Autodesk Inventor part; units mm, degrees
ref_plane "YZ Plane" through (0, 0, 0) normal (1, 0, 0) x (0, 1, 0)
ref_plane "XZ Plane" through (0, 0, 0) normal (0, 1, 0) x (-1, 0, 0)
ref_plane "XY Plane" through (0, 0, 0) normal (0, 0, 1) x (1, 0, 0)
sketch "Sketch1" plane through (0, 0, 0) normal (0, 1, 0) x (-1, 0, 0)
  line L0 (-25, -30) -> (25, -30)
  line L1 (25, -30) -> (25, 30)
  line L2 (25, 30) -> (-25, 30)
  line L3 (-25, 30) -> (-25, -30)
  line L4 (-25, -30) -> (25, 30) construction
  line L5 (25, -30) -> (-25, 30) construction
  point P0 (0, 0)
  dimension "d0" = 50
  dimension "d1" = 60
extrude "Extrusion1" add sketch "Sketch1" along normal blind 53
sketch "Sketch2" plane through (-25, 0, 30) normal (0, 0, 1) x (1, 0, 0)
  line L0 (0, 0) -> (0, 53)
  line L1 (50, 0) -> (50, 53)
  line L2 (0, 53) -> (50, 53)
  line L3 (50, 53) -> (50, 49)
  line L4 (50, 49) -> (0, 49)
  line L5 (0, 49) -> (0, 53)
  line L6 (12.5, 49) -> (37.5, 49)
  line L7 (37.5, 49) -> (37.5, 57)
  line L8 (37.5, 57) -> (12.5, 57)
  line L9 (12.5, 57) -> (12.5, 49)
  line L10 (0, 53) -> (50, 53)
  line L11 (12.5, 49) -> (37.5, 57) construction
  line L12 (37.5, 49) -> (12.5, 57) construction
  line L13 (25, 49) -> (25, 11.5)
  line L14 (46, 11.5) -> (4, 11.5)
  line L15 (4, 11.5) -> (4, 49)
  line L16 (4, 49) -> (46, 49)
  line L17 (46, 49) -> (46, 11.5)
  line L18 (46, 11.5) -> (4, 49) construction
  line L19 (4, 11.5) -> (46, 49) construction
  point P0 (25, 0)
  point P1 (25, 53)
  point P2 (25, 30.25)
  point P3 (37.5, 49)
  point P4 (37.5, 53)
  point P5 (12.5, 53)
  point P6 (12.5, 49)
  dimension "d4" = 4
  dimension "d5" = 25
  dimension "d6" = 8
  dimension "d7" = 37.5
  dimension "d8" = 42
extrude "Extrusion2" cut sketch "Sketch2" against normal blind 51 contours L4 L13 L14 L15 | L2 L7 L4 L9 | L4 L17 L14 L13
sketch "Sketch3" plane through (25, 0, 30) normal (1, 0, 0) x (0, 0, -1)
  line L0 (30, 0) -> (12.5, 0)
  line L1 (12.5, 0) -> (47.5, 0)
  line L2 (0, 0) -> (60, 0)
  circle A0 centre (12.5, 0) radius 7.5
  circle A1 centre (47.5, 0) radius 7.5
  point P0 (55, 0)
  point P1 (40, 0)
  point P2 (20, 0)
  point P3 (5, 0)
  dimension "d11" = 17.5
  dimension "d12" = 35
  dimension "d13" = 15
  dimension "d14" = 15
extrude "Extrusion3" cut sketch "Sketch3" against normal blind 37 contours L0 L2 A0 | A1 L2 L1 picked at (17.141, 1.7601) picked at (45.1933, 4.395)
extrude "Extrusion4" add sketch "Sketch3" against normal blind 13 contours L0 L2 A0 | A1 L2 L1 picked at (17.141, 1.7601) picked at (45.1933, 4.395)
fillet "Fillet1" radius 4 11 edges at (25, 53, 0) (-25, 53, 0) (25, 26.5, 30) (-25, 26.5, 30) (25, 0, 0) (25, 26.5, -30) (0, 53, -30) (-25, 26.5, -30) (-25, 0, 0) (0, 0, 30) (0, 0, -30)
sketch "Sketch4" plane through (-25, 4, 26) normal (-1, 0, 0) x (0, 0, 1)
  line L0 (-35, -15) -> (-17, -15)
  line L1 (-17, -15) -> (-17, 7)
  line L2 (-17, 7) -> (-35, 7)
  line L3 (-35, 7) -> (-35, -15)
  line L4 (-35, -15) -> (-17, 7) construction
  line L5 (-17, -15) -> (-35, 7) construction
  point P0 (-26, -4)
  dimension "d20" = 18
  dimension "d21" = 22
extrude "Extrusion5" cut sketch "Sketch4" against normal through all
sketch "Sketch5" plane through (0, 53, 0) normal (0, 1, 0) x (1, 0, 0)
  line L0 (-12.5, 21) -> (12.5, 21)
  line L1 (0, 21) -> (0, -21)
  line L2 (0, 21) -> (42, 21) construction
  line L3 (15.5, 15.5) -> (-15.5, 15.5)
  line L4 (-15.5, 15.5) -> (-15.5, -15.5)
  line L5 (-15.5, -15.5) -> (15.5, -15.5)
  line L6 (15.5, -15.5) -> (15.5, 15.5)
  line L7 (15.5, 15.5) -> (-15.5, -15.5) construction
  line L8 (-15.5, 15.5) -> (15.5, -15.5) construction
  point P0 (0, 0)
  dimension "d24" = 42
  dimension "d25" = 90
  dimension "d26" = 31
  dimension "d27" = 31
hole "Hole1" at (15.5, 53, 15.5) at (15.5, 53, -15.5) at (-15.5, 53, -15.5) at (-15.5, 53, 15.5) direction (0, -1, 0) diameter 2.4 depth 4 countersink diameter 4 countersink angle 90
properties part number "Joint_Bearings"
Can you work these out from the model? Positions are in its coordinate system, mm. A direction names the side the tool comes from. Round coordinates to 2 decimals unless told otherwise and drop trailing zeros. Loops run counter-clockwise (first coordinate to the right, second up) from the corner with the lowest first, then second, coordinate; pieces in that order, holes last. Notation, with made-up numbers: (47.25, 26) - (69.25, 26) arc R24 cw to (69.25, 40) - close; hole circle Ø7 at (32, 29). An arc over 180 degrees is marked (long way). Use CSV: the item, a comma, the result in double quotes. Start each with the question number.
1) If we section it at D-D on x = 10: Write out the boundary of the cut face in (y, z).
2) If we section it at C-C on z = -15.5: Count the separate pieces of the cut face and the enclosed holes in it, plus the area to 3 significant figures.
3) Please list where these lines run through material, in increasing order: probe 1 along Y at (x, z) = (-16.5, 12.5); probe 2 along Z at (x, y) = (11, 8); probe 3 along X at (y, z) = (33, -0.5). Write a range as [from, to].
4) We'd pull the mould along Z, two halves only. Please class faces 1 (the cylindrical face through (23.859, 1.203, -17.619)), 2 (the flat face through (-12, 3, -17)), 3 (the flat face through (0, 26, -30)): released by +Z, released by -Z, zero draft, split by the parting line, or undercut.
5) For pin 1 Ø3 at (x, z) = (15.5, 15.5) entering from +Y; pin 2 Ø4.5 at (y, z) = (51, -6) entering from +X; pin 3 Ø1 at (x, z) = (8, 18.5) entering from +Y; pin 4 Ø5.5 at (x, z) = (9.5, 2.5) entering from -Y, each with a flat end and sliding along its axis, tell me the tip position at first contact or that it passes through.
6) If we section it at A-A on x = -15.5: Write out the boundary of the cut face in (y, z).
7) For faces 4 (the flat face through (-12.5, 51, 5)), 5 (the flat face through (-25, 26, 0)), 6 (the flat face through (14, 53, 2)), 7 (the flat face through (17, 49, 5)), 8 (the flat face through (12, 3, -17)), which set-ups out of +Z, -Z, +X, -X, +Y, -Y let a thin tool reach every point of the face, with its end or its side?
Geometry results:
1,outline,"(0, -26) arc R4 ccw to (4, -30) - (49, -30) arc R4 ccw to (53, -26) - (53, -21) - (11.5, -21) - (11.5, 30) - (4, 30) arc R4 ccw to (0, 26) - (0, 25) arc R7.5 cw to (0, 10) - (0, 9) - (11, 9) - (11, -9) - (0, -9) - (0, -10) arc R7.5 cw to (0, -25) - close"
2,separate pieces,"3"
2,enclosed holes,"0"
2,area,"767 mm2"
3,probe 1,"y = [0, 11.5], [49, 53]"
3,probe 2,"z = [-30, -9], [9, 30]"
3,probe 3,"x = [-25, -21], [21, 25]"
4,face 1,"zero draft"
4,face 2,"undercut"
4,face 3,"released by -Z"
5,pin 1,"stops at y = 52.5"
5,pin 2,"stops at x = 25"
5,pin 3,"stops at y = 11.5"
5,pin 4,"stops at y = 11"
6,outline,"(0, -26) arc R4 ccw to (4, -30) - (49, -30) arc R4 ccw to (53, -26) - (53, -17.5) - (52.2, -16.7) - (49, -16.7) - (49, -21) - (11.5, -21) - (11.5, 30) - (4, 30) arc R4 ccw to (0, 26) - (0, 9) - (11, 9) - (11, -9) - (0, -9) - close; (49, -14.3) - (52.2, -14.3) - (53, -13.5) - (53, 13.5) - (52.2, 14.3) - (49, 14.3) - close; (49, 16.7) - (52.2, 16.7) - (53, 17.5) - (53, 30) - (49, 30) - close"
7,face 4,"+Z, +Y"
7,face 5,"+Z, -Z, -X, +Y, -Y"
7,face 6,"+Z, -Z, +X, -X, +Y"
7,face 7,"+Z"
7,face 8,"-Y"
